from build123d import *

# Parameters (mm, degrees)
SKETCH_1_W               = 31.500375693
SKETCH_1_H               = 27.5
EXTRUDE_1_DEPTH          = 18.8
SKETCH_2_W               = 0.007172267
SKETCH_2_H               = 21.5
CUT_EXTRUDE_1_DEPTH      = 18.8
SKETCH_3_W               = 30.5
SKETCH_3_H               = 23.5
EXTRUDE_2_DEPTH          = 1.7
SKETCH_4_W               = 28.5
SKETCH_4_H               = 21.5
CUT_EXTRUDE_2_DEPTH      = 12.2
SKETCH_5_W               = 15.8
SKETCH_5_H               = 15.8
EXTRUDE_3_DEPTH          = 0.8
CUT_EXTRUDE_3_DEPTH      = 6.3
SKETCH_7_W               = 14.2
SKETCH_7_H               = 14.2
CUT_EXTRUDE_4_DEPTH      = 0.8
SKETCH_8_W               = 12
SKETCH_8_H               = 12
CUT_EXTRUDE_5_DEPTH      = 26.276152686
CUT_EXTRUDE_6_REACH      = 39.211
HOLE_WIZARD_M2_5_1_D     = 2.85
HOLE_WIZARD_M2_5_1_DEPTH = 5.5
FILLET_1_R               = 2
FILLET_2_R               = 0.5
FILLET_3_R               = 1


with BuildPart() as part:
    # 草图1 → 凸台-拉伸1 (new body)
    with BuildSketch(Plane(origin=(0, 19.5, 0), x_dir=(1, 0, 0), z_dir=(0, 1, 0))):
        with Locations((0.003586134, 0)):
            Rectangle(SKETCH_1_W, SKETCH_1_H)
    extrude(amount=-EXTRUDE_1_DEPTH)

    # 草图2 → 切除-拉伸1 (cut)
    with BuildSketch(Plane.XZ.offset(-0.7)):
        with Locations((15.750187847, 0)):
            Rectangle(SKETCH_2_W, SKETCH_2_H)
    extrude(amount=-CUT_EXTRUDE_1_DEPTH, mode=Mode.SUBTRACT)

    # 草图3 → 凸台-拉伸2 (add)
    with BuildSketch(Plane.XZ.offset(-0.7)):
        Rectangle(SKETCH_3_W, SKETCH_3_H)
    extrude(amount=EXTRUDE_2_DEPTH)

    # 草图4 → 切除-拉伸2 (cut)
    with BuildSketch(Plane.XZ.offset(1)):
        Rectangle(SKETCH_4_W, SKETCH_4_H)
    extrude(amount=-CUT_EXTRUDE_2_DEPTH, mode=Mode.SUBTRACT)

    # 草图5 → 凸台-拉伸3 (add)
    with BuildSketch(Plane.XZ.offset(-11.2)):
        Rectangle(SKETCH_5_W, SKETCH_5_H)
    extrude(amount=EXTRUDE_3_DEPTH)

    # 草图6 → 切除-拉伸3 (cut)
    with BuildSketch(Plane(origin=(0, 19.5, 0), x_dir=(-1, 0, 0), z_dir=(0, 1, 0))):
        with BuildLine():
            Line((-14.25, 7.40625753), (-14.25, -7.40625753))
            ThreePointArc((-14.25, -7.40625753), (-11.590811691, -8.090811691), (-10.90625753, -10.75))
            Line((-10.90625753, -10.75), (10.90625753, -10.75))
            ThreePointArc((10.90625753, -10.75), (11.590811691, -8.090811691), (14.25, -7.40625753))
            Line((14.25, -7.40625753), (14.25, 7.40625753))
            ThreePointArc((14.25, 7.40625753), (11.590811691, 8.090811691), (10.90625753, 10.75))
            Line((10.90625753, 10.75), (-10.90625753, 10.75))
            ThreePointArc((-10.90625753, 10.75), (-11.590811691, 8.090811691), (-14.25, 7.40625753))
        make_face()
    extrude(amount=-CUT_EXTRUDE_3_DEPTH, mode=Mode.SUBTRACT)

    # 草图7 → 切除-拉伸4 (cut)
    with BuildSketch(Plane.XZ.offset(-10.4)):
        Rectangle(SKETCH_7_W, SKETCH_7_H)
    extrude(amount=-CUT_EXTRUDE_4_DEPTH, mode=Mode.SUBTRACT)

    # 草图8 → 切除-拉伸5 (cut, through all)
    with BuildSketch(Plane(origin=(0, 13.2, 0), x_dir=(-1, 0, 0), z_dir=(0, 1, 0))):
        Rectangle(SKETCH_8_W, SKETCH_8_H)
    extrude(amount=-CUT_EXTRUDE_5_DEPTH, mode=Mode.SUBTRACT)

    # 草图9 → 切除-拉伸6 (cut, up to next)
    with BuildSketch(Plane.XY.offset(13.75), mode=Mode.PRIVATE) as cut_extrude_6_sk1:
        Polygon((-4, 17.65), (-4, 15.8), (-3, 14.8), (3, 14.8), (4, 15.8), (4, 17.65), align=None)
    cut_extrude_6_tool1 = extrude(cut_extrude_6_sk1.sketch, amount=-CUT_EXTRUDE_6_REACH, mode=Mode.PRIVATE) & part.part
    add(cut_extrude_6_tool1.solids().sort_by_distance((0, 16.275076, 13.75))[0], mode=Mode.SUBTRACT)

    # M2.5 间隙孔1
    with Locations(Plane(origin=(0, 19.5, 0), x_dir=(1, 0, 0), z_dir=(0, 1, 0))):
        with Locations((13.5, 10), (13.5, -10), (-13.5, -10), (-13.5, 10)):
            Hole(HOLE_WIZARD_M2_5_1_D / 2, depth=HOLE_WIZARD_M2_5_1_DEPTH)

    # 圆角1
    fillet_1_edges = [part.edges().sort_by_distance(p)[0] for p in [
        (15.25, -0.15, -11.75),
        (15.25, -0.15, 11.75),
        (-15.25, -0.15, 11.75),
        (-15.25, -0.15, -11.75),
    ]]
    fillet(fillet_1_edges, radius=FILLET_1_R)

    # 圆角2
    fillet_2_edges = [part.edges().sort_by_distance(p)[0] for p in [
        (-4, 17.65, 12.25),
        (4, 17.65, 12.25),
        (4, 15.8, 12.25),
        (3, 14.8, 12.25),
        (-3, 14.8, 12.25),
        (-4, 15.8, 12.25),
        (-15.25, -1, 0),
        (0, -1, 11.75),
        (15.25, -1, 0),
        (0, -1, -11.75),
        (14.664213562, -1, -11.164213562),
        (-14.664213562, -1, -11.164213562),
        (14.664213562, -1, 11.164213562),
        (-14.664213562, -1, 11.164213562),
    ]]
    fillet(fillet_2_edges, radius=FILLET_2_R)

    # 圆角3
    # the kernel refuses this fillet: 1 mm, written as the material it adds along each edge
    with BuildSketch(Plane(origin=(-14.25, -1, 10.75), x_dir=(1, 0, 0), z_dir=(0, 1, 0))) as fillet_3_piece_1:
        with BuildLine():
            CenterArc((FILLET_3_R, FILLET_3_R), FILLET_3_R, 180, 90)
            Line((0, FILLET_3_R), (0, 0))
            Line((0, 0), (FILLET_3_R, 0))
        make_face()
    extrude(amount=14.7)
    with BuildSketch(Plane(origin=(14.25, -1, 10.75), x_dir=(-1, 0, 0), z_dir=(0, 1, 0)), Plane(origin=(14.25, -1, -10.75), x_dir=(0, 0, 1), z_dir=(0, 1, 0)), Plane(origin=(-14.25, -1, -10.75), x_dir=(1, 0, 0), z_dir=(0, 1, 0))) as fillet_3_piece_2:
        with BuildLine():
            CenterArc((FILLET_3_R, -FILLET_3_R), FILLET_3_R, 90, 90)
            Line((0, -FILLET_3_R), (0, 0))
            Line((0, 0), (FILLET_3_R, 0))
        make_face()
    extrude(amount=14.7)
    with BuildSketch(Plane(origin=(13.5, 13.2, 10), x_dir=(-0.3548034469093428, 0, 0.9349409147434126), z_dir=(0.9349409147434126, 0, 0.3548034469093428))) as fillet_3_piece_3_section:
        with BuildLine():
            CenterArc((2.7 + FILLET_3_R, -FILLET_3_R), FILLET_3_R, 90, 90)
            Line((2.7 + FILLET_3_R, 0), (2.7, 0))
            Line((2.7, 0), (2.7, -FILLET_3_R))
        make_face()
    fillet_3_piece_3 = revolve(axis=Axis((13.5, 13.2, 10), (0, -1, 0)), revolution_arc=228.43720284, mode=Mode.PRIVATE)
    fillet_3_piece_3 = split(fillet_3_piece_3, bisect_by=Plane(origin=(14.25, 13.485154119, 7.889177279), z_dir=(-1, 0, 0)), keep=Keep.TOP, mode=Mode.PRIVATE)
    add(fillet_3_piece_3)
    with BuildSketch(Plane(origin=(-13.40625753, 13.2, 10.75), x_dir=(0, 1, 0), z_dir=(1, 0, 0))) as fillet_3_piece_4_section:
        with BuildLine():
            CenterArc((FILLET_3_R, -FILLET_3_R), FILLET_3_R, 90, 90)
            Line((0, -FILLET_3_R), (0, 0))
            Line((0, 0), (FILLET_3_R, 0))
        make_face()
    fillet_3_piece_4 = extrude(amount=26.81251506, mode=Mode.PRIVATE)
    fillet_3_piece_4 = fillet_3_piece_4 - Plane(origin=(13.5, 14.049901013, 10), x_dir=(-0.9606453592105874, 0, 0.27777777777777996), z_dir=(0, 1, 0)) * Cylinder(2.7, 58, mode=Mode.PRIVATE)
    fillet_3_piece_4 = fillet_3_piece_4 - Plane(origin=(-13.5, 14.049901013, 10), x_dir=(-0.2777777777777764, 0, -0.9606453592105884), z_dir=(0, 1, 0)) * Cylinder(2.7, 58, mode=Mode.PRIVATE)
    add(fillet_3_piece_4)
    with BuildSketch(Plane(origin=(-13.5, 13.2, 10), x_dir=(-0.9349409147434112, 0, -0.35480344690934623), z_dir=(-0.35480344690934623, 0, 0.9349409147434112))) as fillet_3_piece_5_section:
        with BuildLine():
            CenterArc((2.7 + FILLET_3_R, -FILLET_3_R), FILLET_3_R, 90, 90)
            Line((2.7 + FILLET_3_R, 0), (2.7, 0))
            Line((2.7, 0), (2.7, -FILLET_3_R))
        make_face()
    fillet_3_piece_5 = revolve(axis=Axis((-13.5, 13.2, 10), (0, -1, 0)), revolution_arc=228.43720284, mode=Mode.PRIVATE)
    fillet_3_piece_5 = split(fillet_3_piece_5, bisect_by=Plane(origin=(-14.25, 13.485154119, 7.889177279), z_dir=(1, 0, 0)), keep=Keep.TOP, mode=Mode.PRIVATE)
    add(fillet_3_piece_5)
    with BuildSketch(Plane(origin=(-14.25, 13.2, -9.90625753), x_dir=(0, 1, 0), z_dir=(0, 0, 1))) as fillet_3_piece_6_section:
        with BuildLine():
            CenterArc((FILLET_3_R, -FILLET_3_R), FILLET_3_R, 90, 90)
            Line((0, -FILLET_3_R), (0, 0))
            Line((0, 0), (FILLET_3_R, 0))
        make_face()
    fillet_3_piece_6 = extrude(amount=19.81251506, mode=Mode.PRIVATE)
    fillet_3_piece_6 = fillet_3_piece_6 - Plane(origin=(-13.5, 14.049902267, 10), x_dir=(-0.2777777777777764, 0, -0.9606453592105884), z_dir=(0, 1, 0)) * Cylinder(2.7, 44, mode=Mode.PRIVATE)
    fillet_3_piece_6 = fillet_3_piece_6 - Plane(origin=(-13.5, 14.049902267, -10), x_dir=(-1, 0, 0), z_dir=(0, -1, 0)) * Cylinder(1.425, 44, mode=Mode.PRIVATE)
    add(fillet_3_piece_6)
    with BuildSketch(Plane(origin=(-13.5, 13.2, -10), x_dir=(0.35480344690934373, 0, -0.9349409147434123), z_dir=(-0.9349409147434123, 0, -0.35480344690934373))) as fillet_3_piece_7_section:
        with BuildLine():
            CenterArc((2.7 + FILLET_3_R, -FILLET_3_R), FILLET_3_R, 90, 90)
            Line((2.7 + FILLET_3_R, 0), (2.7, 0))
            Line((2.7, 0), (2.7, -FILLET_3_R))
        make_face()
    fillet_3_piece_7 = revolve(axis=Axis((-13.5, 13.2, -10), (0, -1, 0)), revolution_arc=228.43720284, mode=Mode.PRIVATE)
    fillet_3_piece_7 = split(fillet_3_piece_7, bisect_by=Plane(origin=(-14.25, 13.485154119, -7.889177279), z_dir=(1, 0, 0)), keep=Keep.TOP, mode=Mode.PRIVATE)
    add(fillet_3_piece_7)
    with BuildSketch(Plane(origin=(13.40625753, 13.2, -10.75), x_dir=(0, 1, 0), z_dir=(-1, 0, 0))) as fillet_3_piece_8_section:
        with BuildLine():
            CenterArc((FILLET_3_R, -FILLET_3_R), FILLET_3_R, 90, 90)
            Line((0, -FILLET_3_R), (0, 0))
            Line((0, 0), (FILLET_3_R, 0))
        make_face()
    fillet_3_piece_8 = extrude(amount=26.81251506, mode=Mode.PRIVATE)
    fillet_3_piece_8 = fillet_3_piece_8 - Plane(origin=(-13.5, 14.049901014, -10), x_dir=(-1, 0, 0), z_dir=(0, -1, 0)) * Cylinder(1.425, 58, mode=Mode.PRIVATE)
    fillet_3_piece_8 = fillet_3_piece_8 - Plane(origin=(13.5, 14.049901014, -10), x_dir=(-1, 0, 0), z_dir=(0, -1, 0)) * Cylinder(1.425, 58, mode=Mode.PRIVATE)
    add(fillet_3_piece_8)
    with BuildSketch(Plane(origin=(13.5, 13.2, -10), x_dir=(0.9349409147434106, 0, 0.3548034469093482), z_dir=(0.3548034469093482, 0, -0.9349409147434106))) as fillet_3_piece_9_section:
        with BuildLine():
            CenterArc((2.7 + FILLET_3_R, -FILLET_3_R), FILLET_3_R, 90, 90)
            Line((2.7 + FILLET_3_R, 0), (2.7, 0))
            Line((2.7, 0), (2.7, -FILLET_3_R))
        make_face()
    fillet_3_piece_9 = revolve(axis=Axis((13.5, 13.2, -10), (0, -1, 0)), revolution_arc=228.43720284, mode=Mode.PRIVATE)
    fillet_3_piece_9 = split(fillet_3_piece_9, bisect_by=Plane(origin=(14.25, 13.485154119, -7.889177279), z_dir=(-1, 0, 0)), keep=Keep.TOP, mode=Mode.PRIVATE)
    add(fillet_3_piece_9)
    with BuildSketch(Plane(origin=(14.25, 13.2, 9.90625753), x_dir=(0, 1, 0), z_dir=(0, 0, -1))) as fillet_3_piece_10_section:
        with BuildLine():
            CenterArc((FILLET_3_R, -FILLET_3_R), FILLET_3_R, 90, 90)
            Line((0, -FILLET_3_R), (0, 0))
            Line((0, 0), (FILLET_3_R, 0))
        make_face()
    fillet_3_piece_10 = extrude(amount=19.81251506, mode=Mode.PRIVATE)
    fillet_3_piece_10 = fillet_3_piece_10 - Plane(origin=(13.5, 14.049902266, 10), x_dir=(-0.9606453592105874, 0, 0.27777777777777996), z_dir=(0, 1, 0)) * Cylinder(2.7, 44, mode=Mode.PRIVATE)
    fillet_3_piece_10 = fillet_3_piece_10 - Plane(origin=(13.5, 14.049902266, -10), x_dir=(-1, 0, 0), z_dir=(0, -1, 0)) * Cylinder(1.425, 44, mode=Mode.PRIVATE)
    add(fillet_3_piece_10)
    # the kernel refuses this fillet: 1 mm, written as the material it takes off along each edge
    with BuildSketch(Plane(origin=(15.75377398, 22, -13.75), x_dir=(0, 0, 1), z_dir=(0, -1, 0)), Plane(origin=(15.75377398, 22, 13.75), x_dir=(-1, 0, 0), z_dir=(0, -1, 0)), Plane(origin=(-15.746601713, 22, -13.75), x_dir=(1, 0, 0), z_dir=(0, -1, 0))) as fillet_3_2_piece_1:
        with BuildLine():
            CenterArc((FILLET_3_R, FILLET_3_R), FILLET_3_R, 180, 90)
            Line((0, FILLET_3_R), (0, 0))
            Line((0, 0), (FILLET_3_R, 0))
        make_face()
    extrude(amount=23.8, mode=Mode.SUBTRACT)
    with BuildSketch(Plane(origin=(-15.746601713, 22, 13.75), x_dir=(1, 0, 0), z_dir=(0, -1, 0))) as fillet_3_2_piece_2:
        with BuildLine():
            CenterArc((FILLET_3_R, -FILLET_3_R), FILLET_3_R, 90, 90)
            Line((0, -FILLET_3_R), (0, 0))
            Line((0, 0), (FILLET_3_R, 0))
        make_face()
    extrude(amount=23.8, mode=Mode.SUBTRACT)


solid = part.part
For this review, take the finished solid that the model builds, in its own axes (mm). A direction names the side the tool comes from. Round coordinates to 2 decimals unless told otherwise and drop trailing zeros. Order: outer loops, then holes, each group sorted by start corner. A loop starts at its lowest first (then second) coordinate and runs counter-clockwise, first axis right, second up. Notation, with made-up numbers: (68, 27) -> (87, 27) arc R28 cw to (87, 60) -> close; hole circle Ø7 at (-18, 88.5). An arc over 180 degrees is marked (long way). Write item = value, one per line. Start each with the question number.
1) The part is to be moulded in two halves that separate along X. For faces 1 (the face through (-0.153, 13.501, 10.465)), 2 (the face through (0, 0, 11.75)), 3 (the face through (15.754, 10, -12)), say which applies: +X half, -X half, draft (parallel to the pull), parting line (faces both ways), or undercut.
2) Insertion check: pin 1 (6 mm diameter, centred on x = 10, z = 4, fed in from -Y); pin 2 (3 mm diameter, centred on y = 3, z = -5, fed in from +X); pin 3 (1.3 mm diameter, centred on x = -2, y = 0, fed in from -Z). Each pin has a flat end and moves straight along its axis. Give the tip position at first contact, or say it passes through.
3) Take a section at C-C on y = 18.25. State the section outline as (x, z) points (3 decimals).
4) Tool access review of faces 4 (the face through (0, 12, 6)), 5 (the face through (14.68, 0.09, -11.15)), 6 (the face through (-7.1, 11, 0)), 7 (the face through (-15.25, 0, 0)), 8 (the face through (-14.816, 16.712, -9.454)): name each direction out of +Z, -Z, +X, -X, +Y, -Y from which nothing blocks a thin tool from reaching the whole face with its end or side.
5) To check wall thickness, follow line 1 (Z direction, x = -13.5, y = 15.9) (3 decimals); line 2 (X direction, y = 17.75, z = -10) (3 decimals); line 3 (X direction, y = 0.25, z = 3.25). State the ranges of each line that lie inside material, in increasing order. Write a range as from..to.
Verdict:
q1.face_1 = undercut
q1.face_2 = draft
q1.face_3 = +X half
q2.pin_1 = 10.4
q2.pin_2 = 15.75
q2.pin_3 = -11.75
q3.outline = (-15.747, -12.75) arc R1 ccw to (-14.747, -13.75) -> (14.754, -13.75) arc R1 ccw to (15.754, -12.75) -> (15.754, -10.75) -> (15.747, -10.75) -> (15.747, 10.75) -> (15.754, 10.75) -> (15.754, 12.75) arc R1 ccw to (14.754, 13.75) -> (-14.747, 13.75) arc R1 ccw to (-15.747, 12.75) -> close; hole circle Ø2.85 at (-13.5, -10); hole circle Ø2.85 at (-13.5, 10); hole (-14.25, -7.406) arc R2.7 cw to (-10.906, -10.75) -> (10.906, -10.75) arc R2.7 cw to (14.25, -7.406) -> (14.25, 7.406) arc R2.7 cw to (10.906, 10.75) -> (-10.906, 10.75) arc R2.7 cw to (-14.25, 7.406) -> close; hole circle Ø2.85 at (13.5, -10); hole circle Ø2.85 at (13.5, 10)
q4.face_4 = +Y, -Y
q4.face_5 = -Z, +X, -Y
q4.face_6 = -Y
q4.face_7 = +Z, -Z, -X, -Y
q4.face_8 = +Y
q5.line_1 = -13.75..-11.425, -8.575..-7.3, 7.3..8.575, 11.425..13.75
q5.line_2 = -15.747..-14.925, -12.075..-10.8, 10.8..12.075, 14.925..15.747
q5.line_3 = -15.25..-14.25, 14.25..15.25
